Work out the finished part from the listing and answer in its coordinate system (mm). A direction names the side the tool comes from. Coordinates: 2 decimals unless noted, no trailing zeros. Write each loop counter-clockwise with the first axis right and the second up, starting at its lowest first coordinate (ties: lowest second). Pieces come first, ordered by that corner, then holes. Notation, with made-up numbers: (51, 18) -> (76, 18) arc R33 cw to (76, 54) -> close; hole circle Ø6 at (-0.5, 38). An arc over 180 degrees is marked (long way). Write each question's results on one line, items separated by ' | '. Start each with the question number.
from build123d import *

# Parameters (mm, degrees)
F0_W     = 958.85
F0_H     = 38.1
F1_DEPTH = 19.05
F0_W_2   = 203.2
F2_W     = 2438.4
F2_H     = 38.1
F3_DEPTH = 19.05


with BuildPart() as f1:
    # F0 (on Top) → F1 (new body)
    with BuildSketch(Plane.XY):
        with Locations((-836.5519275119, 19.05)):
            Rectangle(F0_W, F0_H)
    extrude(amount=F1_DEPTH)



with BuildPart() as f1b:
    # F0 (on Top) → F1, piece 2 (new body)
    with BuildSketch(Plane.XY):
        with Locations((23.8730724881, 19.05)):
            Rectangle(F0_W_2, F0_H)
    extrude(amount=F1_DEPTH)


with BuildPart() as f1c:
    # F0 (on Top) → F1, piece 3 (new body)
    with BuildSketch(Plane.XY):
        with Locations((-217.4269275119, 19.05)):
            Rectangle(F0_W_2, F0_H)
    extrude(amount=F1_DEPTH)


with BuildPart() as f1d:
    # F0 (on Top) → F1, piece 4 (new body)
    with BuildSketch(Plane.XY):
        with Locations((642.9980724881, 19.05)):
            Rectangle(F0_W, F0_H)
    extrude(amount=F1_DEPTH)


with BuildPart() as f1_1:
    add(f1.part)

    add(f1b.part)  # F3 merges F1b

    add(f1c.part)  # F3 merges F1c

    add(f1d.part)  # F3 merges F1d
    # F2 (on face) → F3 (join)
    with BuildSketch(Plane.XY.offset(19.05)):
        with Locations((-96.7769275119, 19.05)):
            Rectangle(F2_W, F2_H)
    extrude(amount=F3_DEPTH)


solid = f1_1.part
1. Find the intervals of material crossed by L1, parallel to X at y = 20, z = 18.5, in increasing order.
2. For faces 4 (the face through (-843, 19, 0)), 5 (the face through (-97, 19, 19.05)), determine the directions among +Z, -Z, +X, -X, +Y, -Y from which every point of the face is accessible in a straight line to the end or side of a thin tool.
3. Find section A-A on z = 8.5. Give the vertices of the cut face in (x, y), and give its area (3 significant figures).
4. Given pin 1 Ø10 at (x, y) = (-835.5, 10.5) entering from -Z; pin 2 Ø19 at (x, y) = (139.5, 14.5) entering from -Z, each flat-ended and moving along its own axis, determine where each tip first touches the part or whether it passes through.
5. Find section B-B on y = 11.5. Give the vertices of the cut face in (x, z), and give its area (3 significant figures).
6. Determine the mould class of faces 1 (the face through (-338, 19, 19.05)), 2 (the face through (-219, 19, 0)), 3 (the face through (-1315.977, 19, 19)) for opening direction X: pulls with the +X half, pulls with the -X half, needs draft (parallel to the pull), parting line crosses it, or undercut.
Ans:
1) L1: x = -1315.98 to -357.13, -319.03 to -115.83, -77.73 to 125.47, 163.57 to 1122.42
2) face 4: -Z, +X, -X, +Y, -Y | face 5: -Z, +Y, -Y
3) outline: (-1315.98, 0) -> (-357.13, 0) -> (-357.13, 38.1) -> (-1315.98, 38.1) -> close; (-319.03, 0) -> (-115.83, 0) -> (-115.83, 38.1) -> (-319.03, 38.1) -> close; (-77.73, 0) -> (125.47, 0) -> (125.47, 38.1) -> (-77.73, 38.1) -> close; (163.57, 0) -> (1122.42, 0) -> (1122.42, 38.1) -> (163.57, 38.1) -> close | area: 88,500 mm²
4) pin 1: stops at z = 0 | pin 2: stops at z = 19.05
5) outline: (-1315.98, 0) -> (-357.13, 0) -> (-357.13, 19.05) -> (-319.03, 19.05) -> (-319.03, 0) -> (-115.83, 0) -> (-115.83, 19.05) -> (-77.73, 19.05) -> (-77.73, 0) -> (125.47, 0) -> (125.47, 19.05) -> (163.57, 19.05) -> (163.57, 0) -> (1122.42, 0) -> (1122.42, 38.1) -> (-1315.98, 38.1) -> close | area: 90,700 mm²
6) face 1: undercut | face 2: needs draft | face 3: pulls with the -X half
